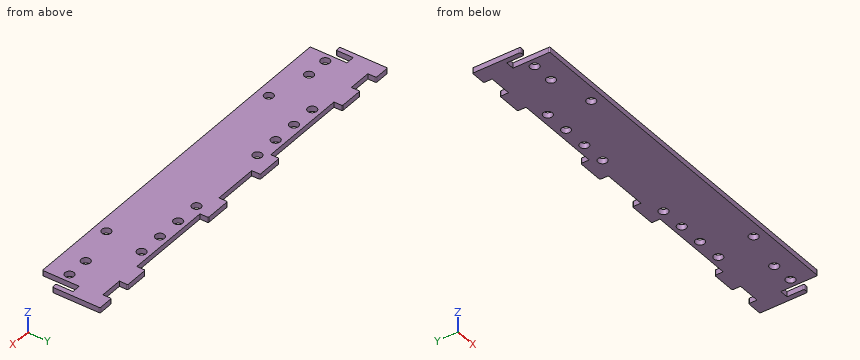
from build123d import *

# Parameters (mm, degrees)
SKETCH41_R                  = 2.5527
BACK_PLATE_EXTRUDE_DEPTH    = 3.0226
SKETCH71_W                  = 8.89
SKETCH71_H                  = 4.7625
SKETCH71_W_2                = 13.79855
SKETCH71_W_3                = 15.09395
BOSS_EXTRUDE26_DEPTH        = 3.0226
SKETCH91_W                  = 4.9022
SKETCH91_H                  = 20.7645
SKETCH91_W_2                = 12.8524
SKETCH91_H_2                = 4.7625
SKETCH91_W_3                = 49.3649
SKETCH91_W_4                = 12.7762
BACK_PLATE_TOLERENCES_DEPTH = 4.0226
FILLET27_R                  = 0.635
FILLET28_R                  = 0.635


with BuildPart() as part:
    # Sketch41 → Back Plate Extrude (new body)
    with BuildSketch(Plane.XY.offset(152.527)):
        Polygon((-104.775, -7.9375), (-104.775, 12.7), (-109.5248, 12.7), (-109.5248, 3.175), (-112.395, 3.175), (-112.395, 25.4), (-104.775, 25.4), (104.775, 25.4), (112.395, 25.4), (112.395, 3.175), (109.5248, 3.175), (109.5248, 12.7), (104.775, 12.7), (104.775, -7.9375), align=None)
        with Locations((-100.0125, 3.9624)):
            Circle(SKETCH41_R, mode=Mode.SUBTRACT)
        with Locations((100.0125, 3.9624)):
            Circle(SKETCH41_R, mode=Mode.SUBTRACT)
        with Locations((23.8252, 20.6375)):
            Circle(SKETCH41_R, mode=Mode.SUBTRACT)
        with Locations((38.1127, 20.6375)):
            Circle(SKETCH41_R, mode=Mode.SUBTRACT)
        with Locations((52.4002, 20.6375)):
            Circle(SKETCH41_R, mode=Mode.SUBTRACT)
        with Locations((66.6877, 20.6375)):
            Circle(SKETCH41_R, mode=Mode.SUBTRACT)
        with Locations((-66.6877, 20.6375)):
            Circle(SKETCH41_R, mode=Mode.SUBTRACT)
        with Locations((-52.4002, 20.6375)):
            Circle(SKETCH41_R, mode=Mode.SUBTRACT)
        with Locations((-38.1127, 20.6375)):
            Circle(SKETCH41_R, mode=Mode.SUBTRACT)
        with Locations((-23.8252, 20.6375)):
            Circle(SKETCH41_R, mode=Mode.SUBTRACT)
        with Locations((-87.3125, 3.9624)):
            Circle(SKETCH41_R, mode=Mode.SUBTRACT)
        with Locations((87.3125, 3.9624)):
            Circle(SKETCH41_R, mode=Mode.SUBTRACT)
        with Locations((-63.5, -1.5875)):
            Circle(SKETCH41_R, mode=Mode.SUBTRACT)
        with Locations((63.5, -1.5875)):
            Circle(SKETCH41_R, mode=Mode.SUBTRACT)
    extrude(amount=BACK_PLATE_EXTRUDE_DEPTH)

    # Sketch71 → Boss-Extrude26 (add, through all)
    with BuildSketch(Plane.XY.offset(155.5496)):
        with Locations((-107.95, 27.78125)):
            Rectangle(SKETCH71_W, SKETCH71_H)
        with Locations((-83.905725, 27.78125)):
            Rectangle(SKETCH71_W_2, SKETCH71_H)
        with Locations((-20.246975, 27.78125)):
            Rectangle(SKETCH71_W_3, SKETCH71_H)
    boss_extrude26 = extrude(amount=-BOSS_EXTRUDE26_DEPTH)

    # Mirror23: Boss-Extrude26 across plane
    add(boss_extrude26.mirror(Plane(origin=(0, 0, 0), x_dir=(0, 0, 1), z_dir=(1, 0, 0))))

    # Sketch91 → Back Plate Tolerences (cut, through all)
    with BuildSketch(Plane(origin=(0, 0, 152.527), x_dir=(-1, 0, 0), z_dir=(0, 0, -1))):
        with Locations((-107.1499, 2.44475)):
            Rectangle(SKETCH91_W, SKETCH91_H)
        with Locations((-97.155, 27.78125)):
            Rectangle(SKETCH91_W_2, SKETCH91_H_2)
        with Locations((-52.4002, 27.78125)):
            Rectangle(SKETCH91_W_3, SKETCH91_H_2)
        with Locations((-6.3881, 27.78125)):
            Rectangle(SKETCH91_W_4, SKETCH91_H_2)
    back_plate_tolerences = extrude(amount=-BACK_PLATE_TOLERENCES_DEPTH, mode=Mode.SUBTRACT)

    # Mirror25: Back Plate Tolerences across plane
    add(back_plate_tolerences.mirror(Plane(origin=(0, 0, 0), x_dir=(0, 0, 1), z_dir=(1, 0, 0))), mode=Mode.SUBTRACT)

    # Fillet27
    fillet27_edges = [part.edges().sort_by_distance(p)[0] for p in [
        (-112.395, 30.1625, 154.0383),
        (112.395, 30.1625, 154.0383),
        (109.601, 3.175, 154.0383),
        (104.6988, -7.9375, 154.0383),
        (-112.395, 3.175, 154.0383),
        (112.395, 3.175, 154.0383),
        (-109.601, 3.175, 154.0383),
        (-104.6988, -7.9375, 154.0383),
    ]]
    fillet(fillet27_edges, radius=FILLET27_R)

    # Fillet28
    fillet28_edges = [part.edges().sort_by_distance(p)[0] for p in [
        (103.5812, 30.1625, 154.0383),
        (90.7288, 30.1625, 154.0383),
        (77.08265, 30.1625, 154.0383),
        (27.71775, 30.1625, 154.0383),
        (12.7762, 30.1625, 154.0383),
        (-103.5812, 30.1625, 154.0383),
        (-90.7288, 30.1625, 154.0383),
        (-27.71775, 30.1625, 154.0383),
        (-77.08265, 30.1625, 154.0383),
        (-12.7762, 30.1625, 154.0383),
    ]]
    fillet(fillet28_edges, radius=FILLET28_R)


solid = part.part
Input: part model. Units: mm. Frame: model coordinates. Coordinates: 2 decimals unless noted, no trailing zeros. Loops run counter-clockwise (first coordinate to the right, second up) from the corner with the lowest first, then second, coordinate; pieces in that order, holes last. Notation, with made-up numbers: (6, 67.25) -> (28, 67.25) arc R31 ccw to (28, 94.25) -> close; hole circle Ø1 at (63, 13.25). An arc over 180 degrees is marked (long way). Write item = value, one per line. Start each with the question number.
Item 1: Cut plane B-B, the plane x = 53. Return loops of the section in (y, z), plus the area to 3 significant figures.
Item 2: Material intervals for line 1 (X direction, y = 28, z = 153.8) (3 decimals); line 2 (X direction, y = 12, z = 153.85) (3 decimals); line 3 (Y direction, x = -63.5, z = 154.65), sorted ascending.
Item 3: First-contact query: P1, Ø0.9, axis at x = 108, z = 154, coming from the -Y side; P2, Ø1.5, axis at x = 44, z = 154.5, coming from the +Y side. Flat tips, straight axial feed; report the tip coordinate or a pass-through.
Item 4: Cut plane D-D, the plane z = 153.6. Count the separate pieces of the cut face and the enclosed holes in it, plus the area to 3 significant figures.
Item 5: Cut plane A-A, the plane y = 9.5. Return loops of the section in (x, z) (3 decimals), plus the area to 3 significant figures.
Item 6: Cut plane C-C, the plane x = -6.5. Return loops of the section in (y, z), plus the area to 3 significant figures.
Ans:
q1.outline = (-7.94, 152.53) -> (18.16, 152.53) -> (18.16, 155.55) -> (-7.94, 155.55) -> close; (23.12, 152.53) -> (25.4, 152.53) -> (25.4, 155.55) -> (23.12, 155.55) -> close
q1.area = 85.8 mm²
q2.line_1 = -112.395 to -103.581, -90.729 to -77.083, -27.718 to -12.776, 12.776 to 27.718, 77.083 to 90.729, 103.581 to 112.395
q2.line_2 = -112.395 to -109.601, -104.699 to 104.699, 109.601 to 112.395
q2.line_3 = -7.94 to -4.14, 0.97 to 25.4
q3.P1 = 12.83
q3.P2 = 25.4
q4.separate_pieces = 1
q4.enclosed_holes = 14
q4.area = 7,300 mm²
q5.outline = (-112.395, 152.527) -> (-109.601, 152.527) -> (-109.601, 155.55) -> (-112.395, 155.55) -> close; (-104.699, 152.527) -> (104.699, 152.527) -> (104.699, 155.55) -> (-104.699, 155.55) -> close; (109.601, 152.527) -> (112.395, 152.527) -> (112.395, 155.55) -> (109.601, 155.55) -> close
q5.area = 650 mm²
q6.outline = (-7.94, 152.53) -> (25.4, 152.53) -> (25.4, 155.55) -> (-7.94, 155.55) -> close
q6.area = 101 mm²
